For this review, take the finished solid that the model builds, in its own axes (mm). A direction names the side the tool comes from. Give positions to 0.01 mm unless a question says otherwise; leave off trailing zeros. Order: outer loops, then holes, each group sorted by start corner. A loop starts at its lowest first (then second) coordinate and runs counter-clockwise, first axis right, second up.
from build123d import *

# Parameters (mm, degrees)
CUT_EXTRUDE1_DEPTH = 2.5


with BuildPart() as part:
    # Sketch1 → Revolve1 (revolve)
    with BuildSketch(Plane.XY, mode=Mode.PRIVATE) as revolve1_sk:
        Polygon((-5, 0), (-5, 3.95), (-4.7, 4.25), (0, 4.25), (0, 2.5), (70, 2.5), (70, 0), align=None)
    revolve(revolve1_sk.sketch.rotate(Axis((-5, 0, 0), (1, 0, 0)), 180), axis=Axis((-5, 0, 0), (1, 0, 0)))

    # Sketch2 → Cut-Extrude1 (cut)
    with BuildSketch(Plane.ZY.offset(5)):
        Polygon((0, 2.309401077), (-2, 1.154700538), (-2, -1.154700538), (0, -2.309401077), (2, -1.154700538), (2, 1.154700538), align=None)
    extrude(amount=-CUT_EXTRUDE1_DEPTH, mode=Mode.SUBTRACT)

    # Sketch3 → Cut-Revolve1 (revolve, cut)
    with BuildSketch(Plane.XY, mode=Mode.PRIVATE) as cut_revolve1_sk:
        Polygon((-2.5, 0), (-2.5, 2), (-1.298278762, 0), align=None)
    revolve(cut_revolve1_sk.sketch.rotate(Axis((-2.5, 0, 0), (1, 0, 0)), 180), axis=Axis((-2.5, 0, 0), (1, 0, 0)), mode=Mode.SUBTRACT)


solid = part.part
1) Clearance check with flat-ended pins moving along their axes: pin 1 (0.5 mm diameter, centred on y = -1, z = 1.5, fed in from -X); pin 2 (3 mm diameter, centred on x = 41.5, z = 3, fed in from +Y); pin 3 (4 mm diameter, centred on x = 44, z = 1.5, fed in from +Y). State where each tip first meets the part, or that it passes through.
Answer sheet:
pin 1: stops at x = -2.5
pin 2: stops at y = 2
pin 3: stops at y = 2.5
2) Draft analysis for pull direction Y (two halves, no side actions). For faces 1 (the face through (-2.317, 0.553, -4.214)), 2 (the face through (70, 0, 0)), 3 (the face through (-4, 0, -2)), state which applies: +Y half, -Y half, draft (parallel to the pull), parting line (faces both ways), or undercut.
Answer sheet:
face 1: parting line
face 2: draft
face 3: undercut
3) To check wall thickness, follow line 1 (X direction, y = -2.75, z = -1.25); line 2 (Y direction, x = 58.5, z = -0.25); line 3 (Y direction, x = 1, z = 1.5). State the ranges of each line that lie inside material, in increasing order.
Answer sheet:
line 1: x = -5 to 0
line 2: y = -2.49 to 2.49
line 3: y = -2 to 2
4) Tool access review of faces 4 (the face through (-5, -2, -1)), 5 (the face through (-4, 0, 2)), 6 (the face through (35.5, 2.5, -0.1)): name each direction out of +Z, -Z, +X, -X, +Y, -Y from which nothing blocks a thin tool from reaching the whole face with its end or side.
Answer sheet:
face 4: +Z, -Z, -X, +Y, -Y
face 5: -X
face 6: +X
5) We need section A-A on x = 26.5. Give the boundary of the cut face in (y, z), then the cut area to 3 significant figures.
Answer sheet:
outline: circle Ø5 at (0, 0)
area: 19.6 mm2
